from build123d import *

# Parameters (mm, degrees)
MODEL_R                  = 8.05
MODEL_W                  = 5
MODEL_H                  = 5
SALIENTE_EXTRUIR1_DEPTH  = 3
CROQUIS3_W               = 3
CROQUIS3_H               = 36.5
SALIENTE_EXTRUIR2_DEPTH  = 15.8
CROQUIS4_R               = 0.75
CROQUIS4_W               = 11.8
CROQUIS4_H               = 22.5
CORTAR_EXTRUIR1_DEPTH    = 3
CROQUIS5_R               = 1.5
CORTAR_EXTRUIR2_DEPTH    = 1
REDONDEO1_R              = 2
REDONDEO1_OF_SIMETR_A1_R = 2
CROQUIS6_W               = 19.999999999
CROQUIS6_H               = 3
SALIENTE_EXTRUIR3_DEPTH  = 8
REDONDEO2_R              = 2
CROQUIS7_R               = 1.5
CORTAR_EXTRUIR3_DEPTH    = 3
CROQUIS8_R               = 2.25
CORTAR_EXTRUIR4_DEPTH    = 1
CROQUIS9_R               = 12
CORTAR_EXTRUIR5_DEPTH    = 1


with BuildPart() as part:
    # Model → Saliente-Extruir1 (new body)
    with BuildSketch(Plane.XY):
        with BuildLine():
            Line((24.527119253, -12.520997464), (24.527119253, -49.020997464))
            Line((24.527119253, -49.020997464), (28.527119253, -49.020997464))
            ThreePointArc((28.527119253, -49.020997464), (29.941332816, -49.606783901), (30.527119253, -51.020997464))
            ThreePointArc((30.527119253, -51.020997464), (31.112905691, -52.435211026), (32.527119253, -53.020997464))
            Line((32.527119253, -53.020997464), (48.698959582, -53.020997464))
            ThreePointArc((48.698959582, -53.020997464), (50.113173145, -53.606783901), (50.698959583, -55.020997464))
            Line((50.698959583, -55.020997464), (50.698959583, -56.020997464))
            Line((50.698959583, -56.020997464), (70.698959582, -56.020997464))
            Line((70.698959582, -56.020997464), (70.698959582, -55.020997464))
            ThreePointArc((70.698959582, -55.020997464), (71.28474602, -53.606783901), (72.698959583, -53.020997464))
            Line((72.698959583, -53.020997464), (88.870799912, -53.020997464))
            ThreePointArc((88.870799912, -53.020997464), (90.285013474, -52.435211026), (90.870799912, -51.020997464))
            ThreePointArc((90.870799912, -51.020997464), (91.456586349, -49.606783901), (92.870799912, -49.020997464))
            Line((92.870799912, -49.020997464), (96.870799912, -49.020997464))
            Line((96.870799912, -49.020997464), (96.870799912, -12.520997464))
            Line((96.870799912, -12.520997464), (92.870799912, -12.520997464))
            ThreePointArc((92.870799912, -12.520997464), (91.456586349, -11.935211026), (90.870799912, -10.520997464))
            Line((90.870799912, -10.520997464), (90.870799912, 1.98809425))
            ThreePointArc((90.870799912, 1.98809425), (90.150187884, 3.221976478), (88.940527152, 3.982547289))
            ThreePointArc((88.940527152, 3.982547289), (82.560153742, 7.972895656), (80.592387516, 15.236499516))
            ThreePointArc((80.592387516, 15.236499516), (73.016137183, 12.831206377), (66.424253692, 8.389126209))
            ThreePointArc((66.424253692, 8.389126209), (62.464845981, 11.66270114), (60.387431279, 16.361376528))
            ThreePointArc((60.387431279, 16.361376528), (55.039384462, 14.426569266), (50.461877073, 11.051438157))
            ThreePointArc((50.461877073, 11.051438157), (49.41482724, 13.546636971), (50.438823204, 16.051385009))
            ThreePointArc((50.438823204, 16.051385009), (43.800023098, 13.634815248), (38.471226177, 8.99613013))
            ThreePointArc((38.471226177, 8.99613013), (37.976525569, 11.673196605), (38.618250464, 14.318872844))
            ThreePointArc((38.618250464, 14.318872844), (33.077419178, 10.94136051), (30.527119253, 4.974420659))
            Line((30.527119253, 4.974420659), (30.527119253, -10.520997464))
            ThreePointArc((30.527119253, -10.520997464), (29.941332816, -11.935211026), (28.527119253, -12.520997464))
            Line((28.527119253, -12.520997464), (24.527119253, -12.520997464))
        make_face()
        with Locations((73.698959582, -7.020997464)):
            Circle(MODEL_R, mode=Mode.SUBTRACT)
        with Locations((47.698959583, -7.020997464)):
            Circle(MODEL_R, mode=Mode.SUBTRACT)
        with Locations((60.698959582, -35.520997464)):
            Rectangle(MODEL_W, MODEL_H, mode=Mode.SUBTRACT)
        with Locations((52.698959582, -35.520997464)):
            Rectangle(MODEL_W, MODEL_H, mode=Mode.SUBTRACT)
        Polygon((57.614023092, -25.177730724), (53.283896073, -27.677730724), (55.783896073, -32.007857743), (60.114023092, -29.507857743), align=None, mode=Mode.SUBTRACT)
        Polygon((68.114023092, -27.677730724), (63.783896073, -25.177730724), (61.283896073, -29.507857743), (65.614023092, -32.007857743), align=None, mode=Mode.SUBTRACT)
        with Locations((68.698959582, -35.520997464)):
            Rectangle(MODEL_W, MODEL_H, mode=Mode.SUBTRACT)
        Polygon((63.783896073, -45.864264204), (68.114023092, -43.364264204), (65.614023092, -39.034137185), (61.283896073, -41.534137185), align=None, mode=Mode.SUBTRACT)
        Polygon((53.283896073, -43.364264203), (57.614023092, -45.864264203), (60.114023092, -41.534137185), (55.783896073, -39.034137185), align=None, mode=Mode.SUBTRACT)
    extrude(amount=SALIENTE_EXTRUIR1_DEPTH)

    # Croquis3 → Saliente-Extruir2 (add)
    with BuildSketch(Plane(origin=(0, 0, 0), x_dir=(-1, 0, 0), z_dir=(0, 0, -1))):
        with Locations((-95.370799912, -30.770997464)):
            Rectangle(CROQUIS3_W, CROQUIS3_H)
    saliente_extruir2 = extrude(amount=SALIENTE_EXTRUIR2_DEPTH)

    # Croquis4 → Cortar-Extruir1 (cut)
    with BuildSketch(Plane(origin=(96.870799912, 0, 0), x_dir=(0, 0, -1), z_dir=(1, 0, 0))):
        with Locations((7.9, -44.420997464)):
            Circle(CROQUIS4_R)
        with Locations((7.9, -17.120997464)):
            Circle(CROQUIS4_R)
        with Locations((7.9, -30.770997464)):
            Rectangle(CROQUIS4_W, CROQUIS4_H)
    cortar_extruir1 = extrude(amount=-CORTAR_EXTRUIR1_DEPTH, mode=Mode.SUBTRACT)

    # Croquis5 → Cortar-Extruir2 (cut)
    with BuildSketch(Plane(origin=(96.870799912, 0, 0), x_dir=(0, 0, -1), z_dir=(1, 0, 0))):
        with Locations((7.9, -17.120997464)):
            Circle(CROQUIS5_R)
        with Locations((7.9, -44.420997464)):
            Circle(CROQUIS5_R)
    cortar_extruir2 = extrude(amount=-CORTAR_EXTRUIR2_DEPTH, mode=Mode.SUBTRACT)

    # Redondeo1
    redondeo1_edges = [part.edges().sort_by_distance(p)[0] for p in [
        (95.370799912, -49.020997464, -15.8),
        (95.370799912, -12.520997464, -15.8),
    ]]
    fillet(redondeo1_edges, radius=REDONDEO1_R)

    # Simetría1: Saliente-Extruir2, Cortar-Extruir1, Cortar-Extruir2 across plane
    add(saliente_extruir2.mirror(Plane(origin=(60.700799912, 0, 0), x_dir=(0, 0, 1), z_dir=(1, 0, 0))))
    add(cortar_extruir1.mirror(Plane(origin=(60.700799912, 0, 0), x_dir=(0, 0, 1), z_dir=(1, 0, 0))), mode=Mode.SUBTRACT)
    add(cortar_extruir2.mirror(Plane(origin=(60.700799912, 0, 0), x_dir=(0, 0, 1), z_dir=(1, 0, 0))), mode=Mode.SUBTRACT)

    # Redondeo1 of Simetría1
    redondeo1_of_simetr_a1_edges = [part.edges().sort_by_distance(p)[0] for p in [
        (26.030799912, -49.020997464, -15.8),
        (26.030799912, -12.520997464, -15.8),
    ]]
    fillet(redondeo1_of_simetr_a1_edges, radius=REDONDEO1_OF_SIMETR_A1_R)

    # Croquis6 → Saliente-Extruir3 (add)
    with BuildSketch(Plane(origin=(0, 0, 0), x_dir=(-1, 0, 0), z_dir=(0, 0, -1))):
        with Locations((-60.698959583, -54.520997464)):
            Rectangle(CROQUIS6_W, CROQUIS6_H)
    extrude(amount=SALIENTE_EXTRUIR3_DEPTH)

    # Redondeo2
    redondeo2_edges = [part.edges().sort_by_distance(p)[0] for p in [
        (50.698959583, -54.520997464, -8),
        (70.698959582, -54.520997464, -8),
    ]]
    fillet(redondeo2_edges, radius=REDONDEO2_R)

    # Croquis7 → Cortar-Extruir3 (cut)
    with BuildSketch(Plane(origin=(0, -53.020997464, 0), x_dir=(1, 0, 0), z_dir=(0, 1, 0))):
        with Locations((66.698959583, 3.5)):
            Circle(CROQUIS7_R)
        with Locations((54.698959582, 3.5)):
            Circle(CROQUIS7_R)
    extrude(amount=-CORTAR_EXTRUIR3_DEPTH, mode=Mode.SUBTRACT)

    # Croquis8 → Cortar-Extruir4 (cut)
    with BuildSketch(Plane(origin=(0, -53.020997464, 0), x_dir=(1, 0, 0), z_dir=(0, 1, 0))):
        with Locations((66.698959583, 3.5)):
            Circle(CROQUIS8_R)
        with Locations((54.698959582, 3.5)):
            Circle(CROQUIS8_R)
    extrude(amount=-CORTAR_EXTRUIR4_DEPTH, mode=Mode.SUBTRACT)

    # Croquis9 → Cortar-Extruir5 (cut)
    with BuildSketch(Plane(origin=(0, 0, 0), x_dir=(-1, 0, 0), z_dir=(0, 0, -1))):
        with Locations((-60.698959582, -35.520997464)):
            Circle(CROQUIS9_R)
    extrude(amount=-CORTAR_EXTRUIR5_DEPTH, mode=Mode.SUBTRACT)


solid = part.part
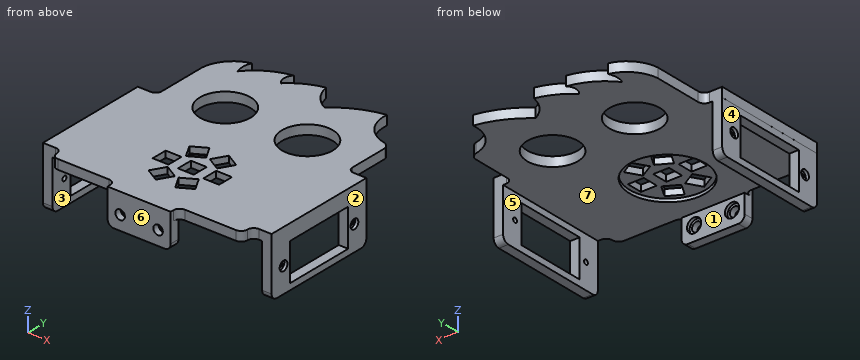
Geometry: final body of the model. Coordinates: model frame, mm. Face numbers are marked on the shaded views. A direction names the side the tool comes from. Coordinates: 2 decimals unless noted, no trailing zeros. Order: outer loops, then holes, each group sorted by start corner. A loop starts at its lowest first (then second) coordinate and runs counter-clockwise, first axis right, second up. Notation, with made-up numbers: M 6,88 L 27,88 A25 cw 27,121 Z; hole C 54.5,70 d3. An arc over 180 degrees is marked long. One line per question, with ' | ' between items. Start each with the question number.
Item 1: Draft query along X for the marked faces 4, 5, 6 and 7. Return one class per face: released by +X, released by -X, zero draft, split by the parting line, or undercut.
Item 2: Cut plane D-D, the plane x = 36.5. Return the cut outline in (y, z), then the cut area to 3 significant figures.
Item 3: Set-up query: the marked faces 1, 2 and 3. Return all of +Z, -Z, +X, -X, +Y, -Y with unobstructed straight access to the full face (end or side cutting, diameter ignored); none if empty.
Item 4: Ray query, probe 1 along Y at (x, z) = (26.05, -7.9); probe 2 along X at (y, z) = (-55.45, -3.5); probe 3 along X at (y, z) = (-26, -1.5). Return the intervals inside material, ascending. Write a range as [from, to].
Item 5: Cut plane A-A, the plane y = -40. Count the separate pieces of the cut face and the enclosed holes in it, then the cut area to 3 significant figures.
Item 6: Pin query (flat end, axial travel): pin 1 Ø8 at (x, y) = (34, -47.5) entering from -Z; pin 2 Ø2.5 at (x, z) = (95.5, -9) entering from -Y; pin 3 Ø5 at (x, z) = (55, -3) entering from +Y; pin 4 Ø4 at (x, z) = (36.5, -3.5) entering from -Y. Return the tip coordinate at first contact, or that it passes through.
Item 7: Cut plane C-C, the plane x = 92. Return the cut outline in (y, z).
A:
1) face 4: released by -X | face 5: undercut | face 6: zero draft | face 7: undercut
2) outline: M -53.02,0 L 13.56,0 L 13.56,3 L -53.02,3 Z | area: 200 mm2
3) face 1: -Z, +X, -X, +Y | face 2: +Z, -Z, +X, +Y, -Y | face 3: -Z, +Y, -Y
4) probe 1: y = [-49.02, -45.17], [-43.67, -42.02], [-19.52, -17.87], [-16.37, -12.52] | probe 2: x = [50.7, 53.2], [56.2, 65.2], [68.2, 70.7] | probe 3: x = [24.53, 27.53], [93.87, 96.87]
5) separate pieces: 5 | enclosed holes: 0 | area: 210 mm2
6) pin 1: stops at z = 0 | pin 2: stops at y = -49.02 | pin 3: stops at y = -53.02 | pin 4: passes through
7) outline: M -49.22,0 L -12.32,0 L -12.32,3 L -49.22,3 Z
